Could you check a few things on this model? Use its own coordinates, in mm. A direction names the side the tool comes from. Give positions to 0.01 mm unless a question says otherwise; leave off trailing zeros. Write each loop counter-clockwise with the first axis right and the second up, starting at its lowest first coordinate (ties: lowest second). Pieces come first, ordered by that corner, then holes. Notation, with made-up numbers: (48, 34) - (54, 34) arc R31 ccw to (54, 72) - close; hole circle Ø8 at (41, 24.25). An arc over 180 degrees is marked (long way). Write item = value, one per line.
from build123d import *

# Parameters (mm, degrees)
SKETCH1_W                      = 66.675
SKETCH1_H                      = 34.925
BOSS_EXTRUDE1_DEPTH            = 38.1
SKETCH2_W                      = 47.625
SKETCH2_H                      = 25.4
CUT_EXTRUDE1_DEPTH             = 85.986868471
SKETCH3_W                      = 34.925
SKETCH3_H                      = 31.75
CUT_EXTRUDE2_DEPTH             = 79.753441393
SKETCH4_W                      = 47.625
SKETCH4_H                      = 38.1
CUT_EXTRUDE3_DEPTH             = 62.504101743
F_1_4_20_TAPPED_HOLE1_D        = 5.1054
F_1_4_20_TAPPED_HOLE1_DEPTH    = 9.526
F_8_32_TAPPED_HOLE2_AT_2_COUNT = 2
F_8_32_TAPPED_HOLE2_AT_2_PITCH = 15.875
LPATTERN1_COUNT                = 2
LPATTERN1_PITCH                = 12.7
MIRROR1_COPY_2_D               = 5.1054
MIRROR1_COPY_2_DEPTH           = 9.526


with BuildPart() as part:
    # Sketch1 → Boss-Extrude1 (new, symmetric)
    with BuildSketch(Plane(origin=(0, 0, 0), x_dir=(1, 0, 0), z_dir=(0, 1, 0))):
        Rectangle(SKETCH1_W, SKETCH1_H)
    extrude(amount=BOSS_EXTRUDE1_DEPTH, both=True)

    # Sketch2 → Cut-Extrude1 (cut, through all)
    with BuildSketch(Plane(origin=(0, 38.1, 0), x_dir=(1, 0, 0), z_dir=(0, 1, 0))):
        with Locations((0, -4.7625)):
            Rectangle(SKETCH2_W, SKETCH2_H)
    extrude(amount=-CUT_EXTRUDE1_DEPTH, mode=Mode.SUBTRACT)

    # Sketch3 → Cut-Extrude2 (cut, through all)
    with BuildSketch(Plane(origin=(33.3375, 0, 0), x_dir=(0, 0, -1), z_dir=(1, 0, 0))):
        with Locations((0, -22.225)):
            Rectangle(SKETCH3_W, SKETCH3_H)
    extrude(amount=-CUT_EXTRUDE2_DEPTH, mode=Mode.SUBTRACT)

    # Sketch4 → Cut-Extrude3 (cut, through all)
    with BuildSketch(Plane(origin=(0, 0, -17.4625), x_dir=(-1, 0, 0), z_dir=(0, 0, -1))):
        with Locations((0, -6.35)):
            Rectangle(SKETCH4_W, SKETCH4_H)
    extrude(amount=-CUT_EXTRUDE3_DEPTH, mode=Mode.SUBTRACT)

    # 1/4-20 Tapped Hole1
    with Locations(Plane(origin=(33.3375, 0, 0), x_dir=(0, 0, -1), z_dir=(1, 0, 0))):
        with Locations((-7.9375, 0), (4.7625, 0)):
            f_1_4_20_tapped_hole1 = Hole(F_1_4_20_TAPPED_HOLE1_D / 2, depth=F_1_4_20_TAPPED_HOLE1_DEPTH)

    # Sketch7 → #8-32 Tapped Hole1 (revolve, cut)
    with BuildSketch(Plane(origin=(26.9875, 5.08, 17.4625), x_dir=(0, -1, 0), z_dir=(1, 0, 0))):
        Polygon((0, 0), (0, 13.483806461), (1.7272, 12.446), (1.7272, 0), align=None)
    f_8_32_tapped_hole1 = revolve(axis=Axis((26.9875, 5.08, 23.8125), (0, 0, -1)), mode=Mode.SUBTRACT)

    # Sketch9 → #8-32 Tapped Hole2 (revolve, cut)
    with BuildSketch(Plane(origin=(28.575, 38.1, 4.7625), x_dir=(0, 0, 1), z_dir=(1, 0, 0))):
        Polygon((0, 0), (0, 13.483806461), (1.7272, 12.446), (1.7272, 0), align=None)
    f_8_32_tapped_hole2 = revolve(axis=Axis((28.575, 44.45, 4.7625), (0, -1, 0)), mode=Mode.SUBTRACT)

    # #8-32 Tapped Hole2 at 2: #8-32 Tapped Hole2 ×2
    with Locations(*[(0, 0, -i * F_8_32_TAPPED_HOLE2_AT_2_PITCH) for i in range(1, F_8_32_TAPPED_HOLE2_AT_2_COUNT)]):
        add(f_8_32_tapped_hole2, mode=Mode.SUBTRACT)

    # LPattern1: 1/4-20 Tapped Hole1 ×2
    with Locations(*[(0, i * LPATTERN1_PITCH, 0) for i in range(1, LPATTERN1_COUNT)]):
        add(f_1_4_20_tapped_hole1, mode=Mode.SUBTRACT)

    # Mirror1: 1/4-20 Tapped Hole1, #8-32 Tapped Hole1, #8-32 Tapped Hole2 across plane
    add(f_1_4_20_tapped_hole1.mirror(Plane(origin=(0, 0, 0), x_dir=(0, 0, 1), z_dir=(1, 0, 0))), mode=Mode.SUBTRACT)
    add(f_8_32_tapped_hole1.mirror(Plane(origin=(0, 0, 0), x_dir=(0, 0, 1), z_dir=(1, 0, 0))), mode=Mode.SUBTRACT)
    add(f_8_32_tapped_hole2.mirror(Plane(origin=(0, 0, 0), x_dir=(0, 0, 1), z_dir=(1, 0, 0))), mode=Mode.SUBTRACT)

    # Mirror1 copy 1 sketch → Mirror1 copy 1 (revolve, cut)
    with BuildSketch(Plane(origin=(-28.575, 38.1, -11.1125), x_dir=(0, 0, 1), z_dir=(-1, 0, 0))):
        Polygon((0, 0), (0, -13.483806461), (1.7272, -12.446), (1.7272, 0), align=None)
    revolve(axis=Axis((-28.575, 44.45, -11.1125), (0, 1, 0)), mode=Mode.SUBTRACT)

    # Mirror1 copy 2
    with Locations(Plane(origin=(-33.3375, 12.7, 0), x_dir=(0, 0, -1), z_dir=(-1, 0, 0))):
        with Locations((-7.9375, 0), (4.7625, 0)):
            Hole(MIRROR1_COPY_2_D / 2, depth=MIRROR1_COPY_2_DEPTH)


solid = part.part
1. Which directions (+Z, -Z, +X, -X, +Y, -Y) give clear straight access to the entire face, cutting with the end or side of a thin tool? Please do faces 1 (the face through (26.862, 31.964, -11.337)), 2 (the face through (0, 26, -7.937)), 3 (the face through (0, 12.7, -13)).
Filled sheet:
face_1 = +Y
face_2 = +Z, +Y, -Y
face_3 = +Z, -Z, -Y
2. For pin 1 (2 mm diameter, centred on x = 26.99, y = 5.08, fed in from +Z); pin 2 (20.5 mm diameter, centred on x = 7, y = 28, fed in from +Z); pin 3 (6 mm diameter, centred on x = -12.5, y = 8, fed in from +Z), each with a flat end and sliding along its axis, tell me the tip position at first contact or that it passes through.
Filled sheet:
pin_1 = 4.58
pin_2 = -7.94
pin_3 = through
3. Thinking about a two-plate mould opening in Z: for faces 4 (the face through (-33.338, 16, 0)), 5 (the face through (-29, 16, 17.462)), 6 (the face through (-28.51, 14.25, 5.91)), which applies, pulls with the +Z half, pulls with the -Z half, needs draft (parallel to the pull), parting line crosses it, or undercut?
Filled sheet:
face_4 = needs draft
face_5 = pulls with the +Z half
face_6 = undercut
4. If we section it at D-D, the plane x = 11: Please give me the cut outline in (y, z), and give its area (3 significant figures).
Filled sheet:
outline = (12.7, -17.46) - (38.1, -17.46) - (38.1, -7.94) - (12.7, -7.94) - close
area = 242 mm2
5. If we section it at C-C, the plane y = 16.5: Please give me the cut outline in (x, z), and give its area (3 significant figures).
Filled sheet:
outline = (-33.34, -17.46) - (33.34, -17.46) - (33.34, 17.46) - (23.81, 17.46) - (23.81, -7.94) - (-23.81, -7.94) - (-23.81, 17.46) - (-33.34, 17.46) - close
area = 1,120 mm2
6. If we section it at A-A, the plane y = 0: Please give me the cut outline in (x, z).
Filled sheet:
outline = (-33.34, -17.46) - (-23.81, -17.46) - (-23.81, -7.32) - (-33.34, -7.32) - close; (-33.34, -2.21) - (-23.81, -2.21) - (-23.81, 5.38) - (-33.34, 5.38) - close; (-33.34, 10.49) - (-23.81, 10.49) - (-23.81, 17.46) - (-33.34, 17.46) - close; (23.81, -17.46) - (33.34, -17.46) - (33.34, -7.32) - (23.81, -7.32) - close; (23.81, -2.21) - (33.34, -2.21) - (33.34, 5.38) - (23.81, 5.38) - close; (23.81, 10.49) - (33.34, 10.49) - (33.34, 17.46) - (23.81, 17.46) - close
7. I need wall thicknesses on line 1 (Z direction, x = -27.75, y = 0); line 2 (X direction, y = 5.08, z = 12.75); line 3 (X direction, y = 22.5, z = 5.5). Which ranges of each line are inside material? Lowest first, please.
Filled sheet:
line_1 = -17.46 to -7.32, -2.21 to 5.38, 10.49 to 17.46
line_2 = -33.34 to -28.71, -25.26 to -23.81, 23.81 to 25.26, 28.71 to 33.34
line_3 = -33.34 to -23.81, 23.81 to 33.34
8. If we section it at B-B, the plane z = -5: Please give me the cut outline in (x, y), and give its area (3 significant figures).
Filled sheet:
outline = (-33.34, -6.35) - (-23.81, -6.35) - (-23.81, -2.54) - (-33.34, -2.54) - close; (-33.34, 2.54) - (-23.81, 2.54) - (-23.81, 10.16) - (-33.34, 10.16) - close; (-33.34, 15.24) - (-23.81, 15.24) - (-23.81, 38.1) - (-33.34, 38.1) - close; (23.81, -6.35) - (33.34, -6.35) - (33.34, -2.54) - (23.81, -2.54) - close; (23.81, 2.54) - (33.34, 2.54) - (33.34, 10.16) - (23.81, 10.16) - close; (23.81, 15.24) - (33.34, 15.24) - (33.34, 38.1) - (23.81, 38.1) - close
area = 653 mm2
